```python
from build123d import *

# Parameters (mm, degrees)
SKETCH1_R           = 15
BOSS_EXTRUDE1_DEPTH = 10
SKETCH2_R           = 5
CUT_EXTRUDE1_DEPTH  = 24.452078799
SKETCH3_R           = 2.5
CUT_EXTRUDE2_DEPTH  = 24.452078799
CIRPATTERN1_COUNT   = 6


with BuildPart() as part:
    # Sketch1 → Boss-Extrude1 (new body)
    with BuildSketch(Plane(origin=(0, 0, 0), x_dir=(1, 0, 0), z_dir=(0, 1, 0))):
        with Locations(Location((0, 0, 0), (0, 0, 270))):
            Circle(SKETCH1_R)
    extrude(amount=BOSS_EXTRUDE1_DEPTH)

    # Sketch2 → Cut-Extrude1 (cut, through all)
    with BuildSketch(Plane(origin=(0, 10, 0), x_dir=(1, 0, 0), z_dir=(0, 1, 0))):
        with Locations(Location((0, 0, 0), (0, 0, 270))):
            Circle(SKETCH2_R)
    extrude(amount=-CUT_EXTRUDE1_DEPTH, mode=Mode.SUBTRACT)

    # Sketch3 → Cut-Extrude2 (cut, through all)
    with BuildSketch(Plane(origin=(0, 10, 0), x_dir=(1, 0, 0), z_dir=(0, 1, 0))):
        with Locations(Location((0, 10, 0), (0, 0, 270))):
            Circle(SKETCH3_R)
    cut_extrude2 = extrude(amount=-CUT_EXTRUDE2_DEPTH, mode=Mode.SUBTRACT)

    # CirPattern1: Cut-Extrude2 ×6 about axis
    cirpattern1_axis = Axis((0, 0, 0), (0, 1, 0))
    for i in range(1, CIRPATTERN1_COUNT):
        add(cut_extrude2.rotate(cirpattern1_axis, i * 360 / CIRPATTERN1_COUNT), mode=Mode.SUBTRACT)


solid = part.part
```
Could you check a few things on this model? Use its own coordinates, in mm. Coordinates: 2 decimals unless noted, no trailing zeros. Loops run counter-clockwise (first coordinate to the right, second up) from the corner with the lowest first, then second, coordinate; pieces in that order, holes last.
1) Imagine slicing it at C-C (z = 7). List the corners of the cut face in (x, y) for me, and give its area (3 significant figures).
Reported:
outline: (-13.27, 0) - (-10.16, 0) - (-10.16, 10) - (-13.27, 10) - close; (-7.16, 0) - (7.16, 0) - (7.16, 10) - (-7.16, 10) - close; (10.16, 0) - (13.27, 0) - (13.27, 10) - (10.16, 10) - close
area: 205 mm2
2) Will these pins go through, and if not, where does the flat tip stop? pin 1 Ø8 at (x, z) = (0, -10) entering from -Y; pin 2 Ø1 at (y, z) = (8.5, -4.5) entering from +X; pin 3 Ø1.5 at (y, z) = (7, 9.5) entering from -X; pin 4 Ø4 at (x, y) = (9, 7) entering from +Z.
Reported:
pin 1: stops at y = 0
pin 2: stops at x = 14.46
pin 3: stops at x = -12.18
pin 4: stops at z = 13.27
3) Imagine slicing it at A-A (x = 0). List the corners of the cut face in (y, z) for me, and give its area (3 significant figures).
Reported:
outline: (0, -15) - (10, -15) - (10, -12.5) - (0, -12.5) - close; (0, -7.5) - (10, -7.5) - (10, -5) - (0, -5) - close; (0, 5) - (10, 5) - (10, 7.5) - (0, 7.5) - close; (0, 12.5) - (10, 12.5) - (10, 15) - (0, 15) - close
area: 100 mm2
4) Imagine slicing it at B-B (z = 10.25). List the corners of the cut face in (x, y) for me.
Reported:
outline: (-10.95, 0) - (-2.49, 0) - (-2.49, 10) - (-10.95, 10) - close; (2.49, 0) - (10.95, 0) - (10.95, 10) - (2.49, 10) - close
5) Thinking about a two-plate mould opening in X: for faces 1 (the face through (0.1, 5.1, -12.5)), 2 (the face through (0.66, 4.93, -14.985)), 3 (the face through (4, 10, -4)), which applies, released by +X, released by -X, zero draft, split by the parting line, or undercut?
Reported:
face 1: undercut
face 2: split by the parting line
face 3: zero draft
6) Imagine slicing it at D-D (y = 5.5). List the corners of the cut face in (x, z) for me.
Reported:
outline: circle Ø30 at (0, 0); hole circle Ø5 at (-8.66, -5); hole circle Ø5 at (-8.66, 5); hole circle Ø10 at (0, 0); hole circle Ø5 at (0, -10); hole circle Ø5 at (0, 10); hole circle Ø5 at (8.66, -5); hole circle Ø5 at (8.66, 5)
7) Please list where these lines run through material, in increasing order: line 1 along Z through (x, y) = (-7.75, 0.5); line 2 along X through (y, z) = (8, 5.25); line 3 along Z through (x, y) = (8.25, 4.75).
Reported:
line 1: z = -12.84 to -7.33, -2.67 to 2.67, 7.33 to 12.84
line 2: x = -14.05 to -11.15, -6.17 to 6.17, 11.15 to 14.05
line 3: z = -12.53 to -7.47, -2.53 to 2.53, 7.47 to 12.53
